Can you work these out from the model? Positions are in its coordinate system, mm. Face numbers are marked on the shaded views. A direction names the side the tool comes from. Round coordinates to 2 decimals unless told otherwise and drop trailing zeros. Write each loop counter-clockwise with the first axis right and the second up, starting at its lowest first coordinate (ties: lowest second). Pieces come first, ordered by that corner, then holes. Notation, with made-up numbers: (37, 35) -> (87, 35) arc R14 cw to (87, 55) -> close; hole circle Ø6 at (-31.5, 70.5). An arc over 180 degrees is marked (long way). Write item = value, one per line. Start each with the question number.
1) Imagine slicing it at C-C, the plane z = 15.5. Please give me the cut outline in (x, y).
2) If I drill on line 1 (Y direction, x = 0, z = 1); line 2 (Z direction, x = -32, y = 23); line 3 (Y direction, x = -30, z = 1), over which ranges is the centre line in solid material (lowest first)?
3) Imagine slicing it at A-A, the plane x = 0. Please give me the cut outline in (y, z), then the cut area to 3 significant figures.
4) For the marked faces 1 and 2, which set-ups out of +Z, -Z, +X, -X, +Y, -Y let a thin tool reach every point of the face, with its end or its side?
5) I'm going to push flat-ended pins straight in: pin 1 (3 mm diameter, centred on x = 30, y = 0, fed in from -Z); pin 2 (8 mm diameter, centred on x = -15.5, y = 40, fed in from +Z); pin 3 (1.5 mm diameter, centred on y = -12, z = 18.5, fed in from +X). Where does each tip first touch, or does it pass through?
from build123d import *

# Parameters (mm, degrees)
F0_R     = 55
F1_DEPTH = 5
F2_R     = 10.85
F3_DEPTH = 25
F4_R     = 12.85
F4_R_2   = 10.85
F5_DEPTH = 30
F7_R     = 2
F8_R     = 1.75
F9_DEPTH = 25


# Not quite as in the source:
# - a fillet or chamfer that OpenCascade refuses, or shapes differently, is made with other operations: its cross-section is extruded or revolved along the edge and cut away or added


with BuildPart() as f1:
    # F0 (on Top) → F1 (new body)
    with BuildSketch(Plane.XY):
        Circle(F0_R)
    extrude(amount=F1_DEPTH)

    # F2 (on face) → F3 (cut)
    with BuildSketch(Plane.XY.offset(5)):
        Circle(F2_R)
    extrude(amount=-F3_DEPTH, mode=Mode.SUBTRACT)

    # F4 (on face) → F5 (join)
    with BuildSketch(Plane.XY.offset(5)):
        Circle(F4_R)
        Circle(F4_R_2, mode=Mode.SUBTRACT)
    extrude(amount=F5_DEPTH)

    # F6: fillet of radius 5 on 1 edges, made by hand

    # F6_s1 → F6_t2 (revolve, cut)
    with BuildSketch(Plane.XZ):
        with BuildLine():
            ThreePointArc((12.85, 31), (12.322135955, 33.2360679775), (10.85, 35))
            Line((10.85, 35), (12.85, 35))
            Line((12.85, 35), (12.85, 31))
        make_face()
    revolve(axis=Axis((0, 0, 35), (0, 0, 1)), mode=Mode.SUBTRACT)

    # F7
    f7_edges = [f1.edges().sort_by_distance(p)[0] for p in [
        (-55, 0, 5),
    ]]
    fillet(f7_edges, radius=F7_R)

    # F8 (on face) → F9 (cut)
    with BuildSketch(Plane.XY.offset(5)):
        with Locations((-30, 0)):
            Circle(F8_R)
        with Locations((0, -30)):
            Circle(F8_R)
        with Locations((30, 0)):
            Circle(F8_R)
        with Locations((0, 30)):
            Circle(F8_R)
    extrude(amount=-F9_DEPTH, mode=Mode.SUBTRACT)


solid = f1.part
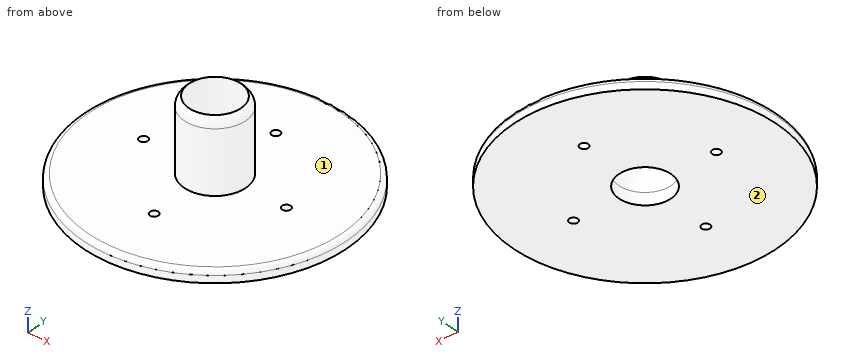
Reported:
q1.outline = circle Ø25.7 at (0, 0); hole circle Ø21.7 at (0, 0)
q2.line_1 = -55 to -31.75, -28.25 to -10.85, 10.85 to 28.25, 31.75 to 55
q2.line_2 = 0 to 5
q2.line_3 = -46.1 to -1.75, 1.75 to 46.1
q3.outline = (-55, 0) -> (-31.75, 0) -> (-31.75, 5) -> (-53, 5) arc R2 ccw to (-55, 3) -> close; (-28.25, 0) -> (-10.85, 0) -> (-10.85, 35) arc R5 ccw to (-12.85, 31) -> (-12.85, 5) -> (-28.25, 5) -> close; (10.85, 0) -> (28.25, 0) -> (28.25, 5) -> (12.85, 5) -> (12.85, 31) arc R5 ccw to (10.85, 35) -> close; (31.75, 0) -> (55, 0) -> (55, 3) arc R2 ccw to (53, 5) -> (31.75, 5) -> close
q3.area = 520 mm²
q4.face_1 = +Z
q4.face_2 = -Z, +X, -X, +Y, -Y
q5.pin_1 = through
q5.pin_2 = 5
q5.pin_3 = 6.21
